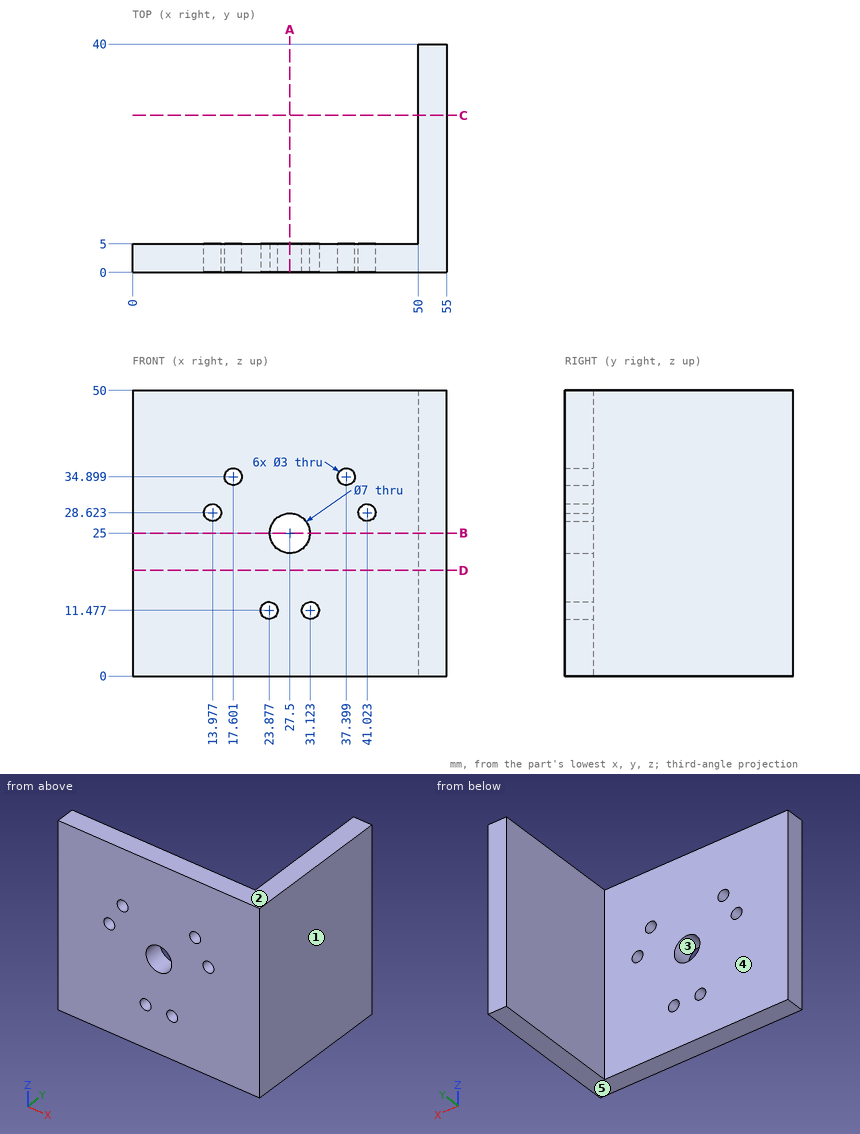
Drawing for the job (mm, zero at the part's lowest x, y, z). A direction names the side the tool comes from. Give positions to 0.01 mm unless a question says otherwise; leave off trailing zeros. Order: outer loops, then holes, each group sorted by start corner. A loop starts at its lowest first (then second) coordinate and runs counter-clockwise, first axis right, second up. Notation, with made-up numbers: M 59.5,-12.5 L 93.5,-12.5 A29 ccw 93.5,19.5 Z; hole C -2.75,36 d2. An arc over 180 degrees is marked long. Write item = value, one per line. Start each with the question number.
(1) Probe L1, parallel to Z at x = 27.5, y = 1.3; L2, parallel to Y at x = 44.5, z = 44; L3, parallel to X at y = 13.5, z = 30. List the from-to ranges inside material, lowest first. Write a range as [from, to].
(2) Which spindle directions (+Z, -Z, +X, -X, +Y, -Y) get a long thin tool onto all of the face, cutting with end or side? Do the marked faces 4 and 5. Say none if no direction does.
(3) Slice it at C-C on y = 27.5. Write the cut outline in (x, z), plus the area to 3 significant figures.
(4) Two-plate mould, pull along Z, no slides. Class the marked faces 1, 2 and 3: released by +Z, released by -Z, zero draft, split by the parting line, or undercut.
(5) Pin check, flat tips, straight feed: pin 1 Ø2.5 at (x, z) = (31.12, 11.48) entering from -Y; pin 2 Ø6 at (x, z) = (28, 35) entering from +Y; pin 3 Ø17.5 at (y, z) = (20.5, 34.5) entering from -X. Stop position of each tip, or through.
(6) Slice it at D-D on z = 18.5. Write the cut outline in (x, y).
(7) Slice it at B-B on z = 25. Write the cut outline in (x, y).
(8) Slice it at A-A on x = 27.5. Write the cut outline in (y, z).
Responses:
q1.L1 = [0, 21.5], [28.5, 50]
q1.L2 = [0, 5]
q1.L3 = [50, 55]
q2.face_4 = +Z, -Z, -X, +Y
q2.face_5 = -Z, +X, -X, +Y, -Y
q3.outline = M 50,0 L 55,0 L 55,50 L 50,50 Z
q3.area = 250 mm2
q4.face_1 = zero draft
q4.face_2 = released by +Z
q4.face_3 = undercut
q5.pin_1 = through
q5.pin_2 = 5
q5.pin_3 = 50
q6.outline = M 0,0 L 55,0 L 55,40 L 50,40 L 50,5 L 0,5 Z
q7.outline = M 0,0 L 24,0 L 24,5 L 0,5 Z; M 31,0 L 55,0 L 55,40 L 50,40 L 50,5 L 31,5 Z
q8.outline = M 0,0 L 5,0 L 5,21.5 L 0,21.5 Z; M 0,28.5 L 5,28.5 L 5,50 L 0,50 Z
